from build123d import *

# Parameters (mm, degrees)
F0_R     = 10.5
F0_R_2   = 10.7
F0_R_3   = 10.9
F0_R_4   = 9.5
F0_R_5   = 8.225
F0_R_6   = 9.7
F0_R_7   = 9.9
F0_R_8   = 8.45
F0_R_9   = 8.65
F0_R_10  = 11.1
F0_R_11  = 11.3
F0_R_12  = 10.1
F0_R_13  = 8.85
F0_R_14  = 9.1
F0_R_15  = 10.3
F0_R_16  = 9.3
F0_R_17  = 7
F0_R_18  = 7.2
F0_R_19  = 7.4
F0_R_20  = 7.6
F0_R_21  = 7.8
F0_R_22  = 8
F1_DEPTH = 25.4


with BuildPart() as f1:
    # F0 (on Front) → F1 (new body)
    with BuildSketch(Plane.XZ):
        Polygon((-18.654427, 46.781804), (-69.954097, 46.781804), (-69.954097, -71.265735), (70.537053, -71.265735), (70.537053, 46.781804), (9.327213, 46.781804), (33.60655, 55.526067), (30.604916, 61.647046), (0.291478, 46.781804), (11.076065, 55.526067), (3.497706, 60.189672), (14.573772, 68.64246), (3.206231, 65.727703), (-4.955082, 75.346395), (-10.493115, 67.476556), (-23.026558, 67.476556), (-13.99082, 60.189672), (-25.35836, 55.526067), (-16.322623, 51.153935), (-44.012789, 59.60672), (-44.012789, 54.65164), align=None)
        with Locations((-49.471106, -53.752262)):
            Circle(F0_R, mode=Mode.SUBTRACT)
        with Locations((-25.496647, -53.752262)):
            Circle(F0_R_2, mode=Mode.SUBTRACT)
        with Locations((-2.283281, -53.752262)):
            Circle(F0_R_3, mode=Mode.SUBTRACT)
        with Locations((-49.090561, -27.304245)):
            Circle(F0_R_4, mode=Mode.SUBTRACT)
        with Locations((-51.882625, 0.810755)):
            Circle(F0_R_5, mode=Mode.SUBTRACT)
        with Locations((-26.828561, -27.304245)):
            Circle(F0_R_6, mode=Mode.SUBTRACT)
        with Locations((-4.947111, -27.304245)):
            Circle(F0_R_7, mode=Mode.SUBTRACT)
        with Locations((-34.102622, 0.810755)):
            Circle(F0_R_8, mode=Mode.SUBTRACT)
        with Locations((-15.156722, 0.810755)):
            Circle(F0_R_9, mode=Mode.SUBTRACT)
        with Locations((22.261996, -53.752262)):
            Circle(F0_R_10, mode=Mode.SUBTRACT)
        with Locations((48.519738, -53.752262)):
            Circle(F0_R_11, mode=Mode.SUBTRACT)
        with Locations((16.934341, -27.304245)):
            Circle(F0_R_12, mode=Mode.SUBTRACT)
        with Locations((3.497706, 0.810755)):
            Circle(F0_R_13, mode=Mode.SUBTRACT)
        with Locations((25.35836, 0.810755)):
            Circle(F0_R_14, mode=Mode.SUBTRACT)
        with Locations((40.718522, -27.304245)):
            Circle(F0_R_15, mode=Mode.SUBTRACT)
        with Locations((47.801968, 0.810755)):
            Circle(F0_R_16, mode=Mode.SUBTRACT)
        with Locations((-52.684705, 30.24547)):
            Circle(F0_R_17, mode=Mode.SUBTRACT)
        with Locations((-34.685574, 30.24547)):
            Circle(F0_R_18, mode=Mode.SUBTRACT)
        with Locations((-16.322624, 30.24547)):
            Circle(F0_R_19, mode=Mode.SUBTRACT)
        with Locations((3.206231, 30.24547)):
            Circle(F0_R_20, mode=Mode.SUBTRACT)
        with Locations((22.152131, 30.24547)):
            Circle(F0_R_21, mode=Mode.SUBTRACT)
        with Locations((42.55541, 30.24547)):
            Circle(F0_R_22, mode=Mode.SUBTRACT)
    extrude(amount=F1_DEPTH)


solid = f1.part
Model file for the job. Use its own axes, mm. A direction names the side the tool comes from. Coordinates: 2 decimals unless noted, no trailing zeros. Order: outer loops, then holes, each group sorted by start corner. A loop starts at its lowest first (then second) coordinate and runs counter-clockwise, first axis right, second up. Notation, with made-up numbers: M 25,85.5 L 61,85.5 A26 ccw 61,104.5 Z; hole C -8.5,64 d11. An arc over 180 degrees is marked long. Return JSON: item names as keys, results as strings.
1. Saw through at B-B (z = -46.5). Give the cut face in (x, y), and give its area (3 significant figures).
Ans:
{"outline": "M -69.95,-25.4 L -57.06,-25.4 L -57.06,0 L -69.95,0 Z; M -41.88,-25.4 L -33.36,-25.4 L -33.36,0 L -41.88,0 Z; M -17.63,-25.4 L -10.42,-25.4 L -10.42,0 L -17.63,0 Z; M 5.85,-25.4 L 13.86,-25.4 L 13.86,0 L 5.85,0 Z; M 30.67,-25.4 L 39.85,-25.4 L 39.85,0 L 30.67,0 Z; M 57.19,-25.4 L 70.54,-25.4 L 70.54,0 L 57.19,0 Z", "area": "1,500 mm^2"}
2. Drill centre lines: probe 1 along Z at (x, y) = (-38, -20.75); probe 2 along Z at (x, y) = (-1.5, -11); probe 3 along Z at (x, y) = (55.5, -21.25). Where is each one in solid material? Low to high.
Ans:
{"probe 1": "-71.27 to -6.69, 8.31 to 23.85, 36.64 to 46.78, 52.79 to 57.77", "probe 2": "-71.27 to -64.62, -42.88 to -36.58, -18.02 to -6.49, 8.11 to 24.28, 36.21 to 71.27", "probe 3": "-71.27 to -62.64, -44.87 to -4.41, 6.03 to 46.78"}
3. Tool access for faces 1 (the face through (-7.09, -12.52, -36.97)), 2 (the face through (8.97, -12.522, 67.205)), 3 (the face through (-17, -13, 67.477)): list every direction of +Z, -Z, +X, -X, +Y, -Y with a clear straight run to the whole face (end or side of a thin tool).
Ans:
{"face 1": "+Y, -Y", "face 2": "+Z, +Y, -Y", "face 3": "+Z, -X, +Y, -Y"}
4. Pull direction X, two halves, no side cores. Call faces 4 (the face through (-1, 0, -13)), 5 (the face through (7.34, -12.522, 57.825)), 6 (the face through (-40.03, -12.52, -24.45)): +X half, -X half, draft (parallel to the pull), parting line (faces both ways), or undercut.
Ans:
{"face 4": "draft", "face 5": "undercut", "face 6": "undercut"}
5. Saw through at D-D (z = -3). Give the cut face in (x, y).
Ans:
{"outline": "M -69.95,-25.4 L -59.17,-25.4 L -59.17,0 L -69.95,0 Z; M -44.59,-25.4 L -41.64,-25.4 L -41.64,0 L -44.59,0 Z; M -26.56,-25.4 L -22.92,-25.4 L -22.92,0 L -26.56,0 Z; M -7.39,-25.4 L -4.49,-25.4 L -4.49,0 L -7.39,0 Z; M 11.49,-25.4 L 17.09,-25.4 L 17.09,0 L 11.49,0 Z; M 33.62,-25.4 L 39.32,-25.4 L 39.32,0 L 33.62,0 Z; M 56.29,-25.4 L 70.54,-25.4 L 70.54,0 L 56.29,0 Z"}
6. Flat gauge pins, fed straight in: pin 1 (21.5 mm diameter, centred on x = -51.88, z = 0.81, fed in from +Y); pin 2 (14 mm diameter, centred on x = 22.15, z = 30.25, fed in from +Y); pin 3 (4 mm diameter, centred on y = -8, z = 58, fed in from -X); pin 4 (6 mm diameter, centred on x = -12.5, y = -20, fed in from +Z). Where does each tip first touch, or does it go through?
Ans:
{"pin 1": "y = 0", "pin 2": "through", "pin 3": "x = -44.01", "pin 4": "z = 68.89"}
7. Saw through at A-A (x = 55). Give the cut face in (y, z).
Ans:
{"outline": "M -25.4,-71.27 L 0,-71.27 L 0,-63.01 L -25.4,-63.01 Z; M -25.4,-44.5 L 0,-44.5 L 0,-5.08 L -25.4,-5.08 Z; M -25.4,6.7 L 0,6.7 L 0,46.78 L -25.4,46.78 Z"}
8. Saw through at C-C (x = -52). Give the cut face in (y, z), and give its area (3 significant figures).
Ans:
{"outline": "M -25.4,-71.27 L 0,-71.27 L 0,-63.94 L -25.4,-63.94 Z; M -25.4,-43.56 L 0,-43.56 L 0,-36.35 L -25.4,-36.35 Z; M -25.4,-18.26 L 0,-18.26 L 0,-7.41 L -25.4,-7.41 Z; M -25.4,9.03 L 0,9.03 L 0,23.28 L -25.4,23.28 Z; M -25.4,37.21 L 0,37.21 L 0,46.78 L -25.4,46.78 Z", "area": "1,250 mm^2"}
